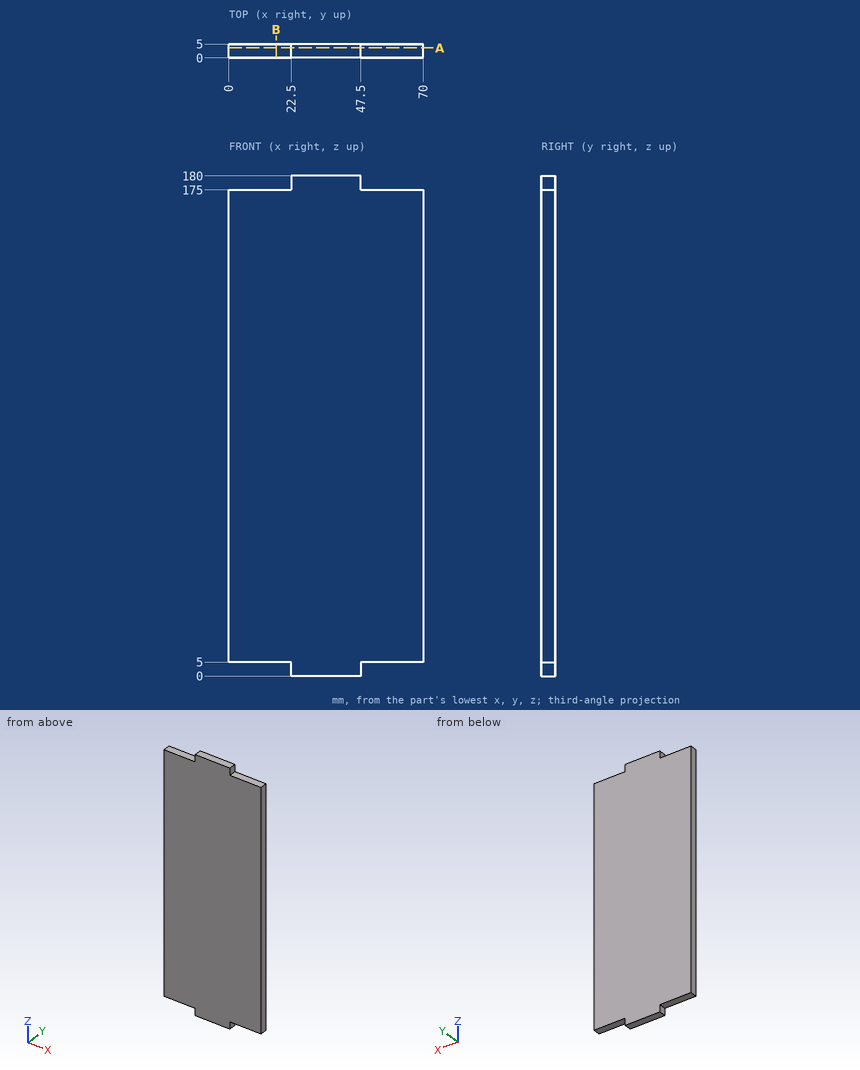
The drawing under review shows one solid part. Ordinate dimensions are in mm from its lowest x, y, z. Round coordinates to 2 decimals unless told otherwise and drop trailing zeros. Write each loop counter-clockwise with the first axis right and the second up, starting at its lowest first coordinate (ties: lowest second). Pieces come first, ordered by that corner, then holes. Notation, with made-up numbers: (33.5, 14.5) - (76.5, 14.5) arc R30 ccw to (76.5, 45.5) - close; hole circle Ø11 at (79, 31.5). An arc over 180 degrees is marked (long way). Use one line per item in the form item = value.
Q1. Consider section A-A (y = 3.6). State the section outline as (x, z) points, and give its area (4 significant figures).
Answer key:
outline = (0, 5) - (22.5, 5) - (22.5, 0) - (47.5, 0) - (47.5, 5) - (70, 5) - (70, 175) - (47.5, 175) - (47.5, 180) - (22.5, 180) - (22.5, 175) - (0, 175) - close
area = 12,150 mm2
Q2. Insertion check: pin 1 Ø1.5 at (x, y) = (8, 2.5) entering from -Z. The pin has a flat end and moves straight along its axis. Give the tip position at first contact, or say it passes through.
Answer key:
pin_1 = 5
Q3. Consider section B-B (x = 17). State the section outline as (y, z) points, and give its area (3 significant figures).
Answer key:
outline = (0, 5) - (5, 5) - (5, 175) - (0, 175) - close
area = 850 mm2
Q4. For line 1 (Z direction, x = 49, y = 0.9), list the stretches that pass through material, from the lowest coordinate up. Write a range as [from, to].
Answer key:
line_1 = [5, 175]
